Build history of the part. All positions in model axes, mm. A direction names the side the tool comes from. Coordinates: 2 decimals unless noted, no trailing zeros. Order: outer loops, then holes, each group sorted by start corner. A loop starts at its lowest first (then second) coordinate and runs counter-clockwise, first axis right, second up. Notation, with made-up numbers: (45.25, 78) - (59.25, 78) arc R10 cw to (59.25, 97) - close; hole circle Ø6 at (-14.5, 46). An arc over 180 degrees is marked (long way). Write each question's results on one line, items separated by ' | '.
from build123d import *

# Parameters (mm, degrees)
BOSS_EXTRUDE1_DEPTH   = 1.5
SKETCH2_W             = 25
SKETCH2_H             = 1.5
BOSS_EXTRUDE2_DEPTH   = 38.5
FILLET1_R             = 2
CUT_EXTRUDE1_DEPTH    = 38.5
M4X0_7_TAPPED_HOLE1_D = 3.3


with BuildPart() as part:
    # Sketch1 → Boss-Extrude1 (new body)
    with BuildSketch(Plane.XY):
        Polygon((-54.090560102, -2.830140877), (70.909439898, -2.830140877), (70.909439898, -67.830140877), (45.909439898, -67.830140877), (45.909439898, -32.830140877), (-54.090560102, -32.830140877), align=None)
    extrude(amount=BOSS_EXTRUDE1_DEPTH)

    # Sketch2 → Boss-Extrude2 (add)
    with BuildSketch(Plane.XY.offset(1.5)):
        with Locations((58.409439898, -67.080140877)):
            Rectangle(SKETCH2_W, SKETCH2_H)
    extrude(amount=BOSS_EXTRUDE2_DEPTH)

    # Fillet1
    fillet1_edges = [part.edges().sort_by_distance(p)[0] for p in [
        (-54.090560102, -2.830140877, 0.75),
        (70.909439898, -2.830140877, 0.75),
        (-54.090560102, -32.830140877, 0.75),
        (45.909439898, -67.080140877, 40),
        (70.909439898, -67.080140877, 40),
    ]]
    fillet(fillet1_edges, radius=FILLET1_R)

    # Sketch3 → Cut-Extrude1 (cut)
    with BuildSketch(Plane.XZ.offset(67.830140877)):
        with BuildLine():
            Line((53.409439898, 32.25), (67.417341478, 32.25))
            ThreePointArc((67.417341478, 32.25), (69.667341478, 30), (67.417341478, 27.75))
            Line((67.417341478, 27.75), (53.409439898, 27.75))
            ThreePointArc((53.409439898, 27.75), (51.159439898, 30), (53.409439898, 32.25))
        make_face()
        with BuildLine():
            Line((67.936439633, 12.75), (53.409439898, 12.75))
            ThreePointArc((53.409439898, 12.75), (51.159439898, 15), (53.409439898, 17.25))
            Line((53.409439898, 17.25), (67.936439633, 17.25))
            ThreePointArc((67.936439633, 17.25), (70.186439633, 15), (67.936439633, 12.75))
        make_face()
    extrude(amount=-CUT_EXTRUDE1_DEPTH, mode=Mode.SUBTRACT)

    # M4x0.7 Tapped Hole1 (through all)
    with Locations(Plane.XY.offset(1.5)):
        with Locations((-44.090560102, -17.830140877), (30.909439898, -17.830140877)):
            Hole(M4X0_7_TAPPED_HOLE1_D / 2)


solid = part.part
1. Band-saw the part on B-B on z = 30. Give the cut face in (x, y).
Solved:
outline: (45.91, -67.83) - (51.16, -67.83) - (51.16, -66.33) - (45.91, -66.33) - close; (69.67, -67.83) - (70.91, -67.83) - (70.91, -66.33) - (69.67, -66.33) - close
2. Drop flat-ended pins along their axis: pin 1 Ø19 at (x, y) = (-21.5, -48.5) entering from +Z; pin 2 Ø20 at (x, z) = (58, 20) entering from +Y; pin 3 Ø1.6 at (x, z) = (1.5, 0.5) entering from -Y. Give the stop position or say it passes through.
Solved:
pin 1: passes through | pin 2: stops at y = -66.33 | pin 3: stops at y = -32.83
3. Band-saw the part on D-D on x = 12. Give the cut face in (y, z).
Solved:
outline: (-32.83, 0) - (-2.83, 0) - (-2.83, 1.5) - (-32.83, 1.5) - close
4. Band-saw the part on A-A on z = 15. Give the cut face in (x, y).
Solved:
outline: (45.91, -67.83) - (51.16, -67.83) - (51.16, -66.33) - (45.91, -66.33) - close; (70.19, -67.83) - (70.91, -67.83) - (70.91, -66.33) - (70.19, -66.33) - close
5. Two-plate mould, pull along Y, no slides. Class faces 4 (the face through (58, -67.83, 20)), 5 (the face through (69.667, -67.091, 30.049)), 6 (the face through (-42.78, -18.83, 0.74)): +Y half, -Y half, draft (parallel to the pull), parting line (faces both ways), or undercut.
Solved:
face 4: -Y half | face 5: draft | face 6: undercut
6. Band-saw the part on C-C on y = -24. Give the cut face in (x, z).
Solved:
outline: (-54.09, 0) - (70.91, 0) - (70.91, 1.5) - (-54.09, 1.5) - close
7. Tool access for faces 1 (the face through (23, -20, 1.5)), 2 (the face through (45.909, -67, 10)), 3 (the face through (51.16, -67.09, 14.95)): list every direction of +Z, -Z, +X, -X, +Y, -Y with a clear straight run to the whole face (end or side of a thin tool).
Solved:
face 1: +Z, +X, -X, +Y | face 2: +Z, -Z, -X, -Y | face 3: +Y, -Y
8. Probe line 1 (Z direction, x = 9, y = -29.5). List the from-to ranges inside material, lowest first.
Solved:
line 1: z = 0 to 1.5
